Could you check a few things on this model? Use its own coordinates, in mm. Face numbers are marked on the shaded views. Round coordinates to 2 decimals unless told otherwise and drop trailing zeros. Loops run counter-clockwise (first coordinate to the right, second up) from the corner with the lowest first, then second, coordinate; pieces in that order, holes last. Notation, with made-up numbers: M 35,63 L 70,63 A28 ccw 70,85 Z; hole C -8,88 d4. An arc over 180 degrees is marked long. Answer in a Markdown table with one row per item.
```python
from build123d import *

# Parameters (mm, degrees)
SKETCH1_R           = 1.25
SKETCH1_R_2         = 4.75
BOSS_EXTRUDE1_DEPTH = 2.5
SKETCH1_9_R         = 6.5
SKETCH1_9_R_2       = 4.75
BOSS_EXTRUDE2_DEPTH = 9
CHAMFER1_SIZE       = 1
CHAMFER1_SIZE2      = 0.577350269
BOSS_EXTRUDE3_DEPTH = 1.25
CIRPATTERN1_COUNT   = 3


with BuildPart() as part:
    # Sketch1 → Boss-Extrude1 (new body)
    with BuildSketch(Plane(origin=(0, 0, 0), x_dir=(1, 0, 0), z_dir=(0, 1, 0))):
        with BuildLine():
            ThreePointArc((7.622629767, -7.943265547), (11.041823898, -6.375), (10.690384636, -2.629758248))
            Line((10.690384636, -2.629758248), (5.629165125, 3.25))
            Line((5.629165125, 3.25), (3.067754869, 10.573023795))
            ThreePointArc((3.067754869, 10.573023795), (0, 12.75), (-3.067754869, 10.573023795))
            Line((-3.067754869, 10.573023795), (-5.629165125, 3.25))
            Line((-5.629165125, 3.25), (-10.690384636, -2.629758248))
            ThreePointArc((-10.690384636, -2.629758248), (-11.041823898, -6.375), (-7.622629767, -7.943265547))
            Line((-7.622629767, -7.943265547), (0, -6.5))
            Line((0, -6.5), (7.622629767, -7.943265547))
        make_face()
        with Locations(Location((-8.227241336, -4.75, 0), (0, 0, 270))):
            Circle(SKETCH1_R, mode=Mode.SUBTRACT)
        with Locations(Location((0, 0, 0), (0, 0, 270))):
            Circle(SKETCH1_R_2, mode=Mode.SUBTRACT)
        with Locations(Location((8.227241336, -4.75, 0), (0, 0, 270))):
            Circle(SKETCH1_R, mode=Mode.SUBTRACT)
        with Locations(Location((0, 9.5, 0), (0, 0, 270))):
            Circle(SKETCH1_R, mode=Mode.SUBTRACT)
    extrude(amount=BOSS_EXTRUDE1_DEPTH)

    # Sketch1_9 → Boss-Extrude2 (add)
    with BuildSketch(Plane(origin=(0, 0, 0), x_dir=(1, 0, 0), z_dir=(0, 1, 0))):
        with Locations(Location((0, 0, 0), (0, 0, 270))):
            Circle(SKETCH1_9_R)
        with Locations(Location((0, 0, 0), (0, 0, 270))):
            Circle(SKETCH1_9_R_2, mode=Mode.SUBTRACT)
    extrude(amount=BOSS_EXTRUDE2_DEPTH)

    # Chamfer1
    chamfer1_edges = [part.edges().sort_by_distance(p)[0] for p in [
        (0, 9, -6.5),
    ]]
    chamfer1_side = [part.faces().sort_by_distance(p)[0] for p in [
        (0, 5.75, -6.5),
    ]]
    chamfer(chamfer1_edges, length=CHAMFER1_SIZE, length2=CHAMFER1_SIZE2, reference=chamfer1_side[0])

    # Sketch1_10 → Boss-Extrude3 (add)
    with BuildSketch(Plane(origin=(0, 0, 0), x_dir=(1, 0, 0), z_dir=(0, 1, 0))):
        with BuildLine():
            ThreePointArc((0, -6.5), (-1.5612495, -6.309714732), (-3.031088913, -5.75))
            Line((-3.031088913, -5.75), (-4.75, -5.75))
            Line((-4.75, -5.75), (-4.75, -7.399363022))
            Line((-4.75, -7.399363022), (0, -6.5))
        make_face()
        with BuildLine():
            Line((3.031088913, -5.75), (-3.031088913, -5.75))
            ThreePointArc((-3.031088913, -5.75), (-1.5612495, -6.309714732), (0, -6.5))
            ThreePointArc((0, -6.5), (1.5612495, -6.309714732), (3.031088913, -5.75))
        make_face()
        with BuildLine():
            Line((4.75, -5.75), (3.031088913, -5.75))
            ThreePointArc((3.031088913, -5.75), (1.5612495, -6.309714732), (0, -6.5))
            Line((0, -6.5), (4.75, -7.399363022))
            Line((4.75, -7.399363022), (4.75, -5.75))
        make_face()
    boss_extrude3 = extrude(amount=-BOSS_EXTRUDE3_DEPTH)

    # CirPattern1: Boss-Extrude3 ×3 about axis
    cirpattern1_axis = Axis((0, 0, 0), (0, 1, 0))
    for i in range(1, CIRPATTERN1_COUNT):
        add(boss_extrude3.rotate(cirpattern1_axis, i * 360 / CIRPATTERN1_COUNT))


solid = part.part
```
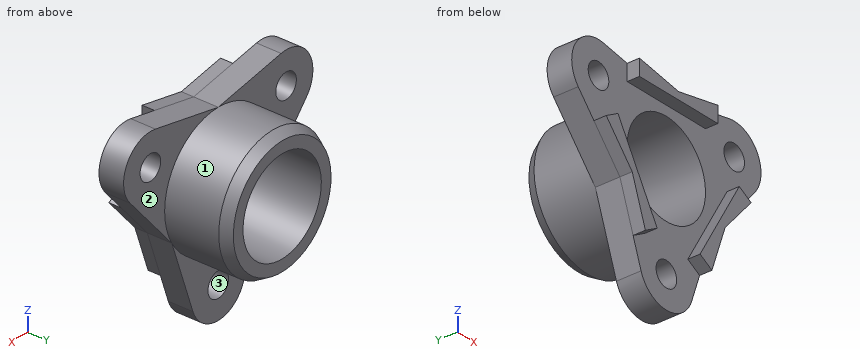
1) I need wall thicknesses on line 1 (X direction, y = -0.5, z = -1.25); line 2 (Y direction, x = -6, z = 6); line 3 (Y direction, x = -4, z = -6.75). Which ranges of each line are inside material? Lowest first, please.
Computed:
| item | result |
|---|---|
| line 1 | x = -7.35 to -5.92, 5.92 to 7.35 |
| line 2 | y = 0 to 2.5 |
| line 3 | y = -1.25 to 2.5 |
2) If we mould it in two halves opening along X, with no side actions, what happens to the marked faces 1, 2 and 3? For each: released by +X, released by -X, zero draft, split by the parting line, or undercut.
Computed:
| item | result |
|---|---|
| face 1 | split by the parting line |
| face 2 | zero draft |
| face 3 | undercut |
3) I want a section at D-D, the plane z = 0. Please give me the cut outline in (x, y), plus the area to 3 significant figures.
Computed:
| item | result |
|---|---|
| outline | M -8.43,-1.25 L -6.64,-1.25 L -6.64,0 L -4.75,0 L -4.75,9 L -5.92,9 L -6.5,8 L -6.5,2.5 L -8.43,2.5 Z; M 4.75,0 L 6.64,0 L 6.64,-1.25 L 8.43,-1.25 L 8.43,2.5 L 6.5,2.5 L 6.5,8 L 5.92,9 L 4.75,9 Z |
| area | 45.0 mm² |
4) I want a section at B-B, the plane y = 5.5. Please give me the cut outline in (x, z).
Computed:
| item | result |
|---|---|
| outline | C 0,0 d13; hole C 0,0 d9.5 |
5) I want a section at A-A, the plane z = -9.5. Please give me the cut outline in (x, y).
Computed:
| item | result |
|---|---|
| outline | M -3.44,0 L -1.25,0 L -1.25,2.5 L -3.44,2.5 Z; M 1.25,0 L 3.44,0 L 3.44,2.5 L 1.25,2.5 Z |
6) Will these pins go through, and if not, where does the flat tip stop? P1, Ø1.5, axis at x = 0, y = 5, coming from the +Z side; P2, Ø5, axis at x = -1.5, z = 2.5, coming from the -Y side; P3, Ø9, axis at x = -6.5, z = 0, coming from the +Y side; P4, Ø2, axis at x = -8.23, z = 4.75, coming from the -Y side.
Computed:
| item | result |
|---|---|
| P1 | stops at z = 6.5 |
| P2 | stops at y = 0 |
| P3 | stops at y = 9 |
| P4 | passes through |
7) I want a section at C-C, the plane x = 9.75. Please give me the cut outline in (y, z), plus the area to 3 significant figures.
Computed:
| item | result |
|---|---|
| outline | M 0,1.54 L 2.5,1.54 L 2.5,7.62 L 0,7.62 Z |
| area | 15.2 mm² |
